```python
from build123d import *

# Parameters (mm, degrees)
F0_R      = 25
F2_DEPTH  = 50
F3_R      = 12.5
F4_DEPTH  = 37.5
F10_D     = 10
F10_DEPTH = 25
F10_TIP   = 3.0043030951
F11_R     = 5
F12_DEPTH = 25


# Not quite as in the source:
# - a feature of the source that left no trace in its solid (it failed there, or was rolled back) is left out


with BuildPart() as f2:
    # F0 (on Top) → F2 (new body)
    with BuildSketch(Plane.XY):
        Circle(F0_R)
    extrude(amount=F2_DEPTH)

    # F3 (on face) → F4 (join)
    with BuildSketch(Plane.XY.offset(50)):
        Circle(F3_R)
    extrude(amount=F4_DEPTH)

    # F10
    with Locations(Plane(origin=(0, 0, 0), x_dir=(1, 0, 0), z_dir=(0, 0, -1))):
        with Locations((0, 0)):
            Hole(F10_D / 2, depth=F10_DEPTH)
            with Locations((0, 0, -(F10_DEPTH + F10_TIP / 2))):  # 118° drill point
                Cone(0, F10_D / 2, F10_TIP, mode=Mode.SUBTRACT)

    # F11 (on face) → F12 (join)
    with BuildSketch(Plane.XY.offset(87.5)):
        Circle(F11_R)
    extrude(amount=F12_DEPTH)


solid = f2.part
```
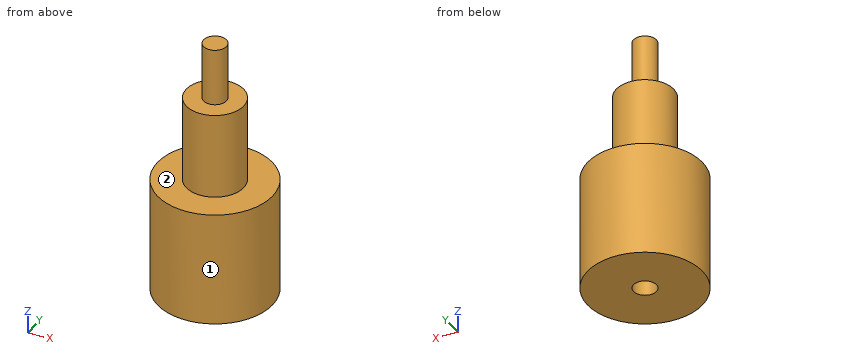
Design review of the part built by this model. Coordinates are the model's own, in mm. Face numbers are marked on the shaded views. A direction names the side the tool comes from. Round coordinates to 2 decimals unless told otherwise and drop trailing zeros. Write each loop counter-clockwise with the first axis right and the second up, starting at its lowest first coordinate (ties: lowest second). Pieces come first, ordered by that corner, then holes. Notation, with made-up numbers: (-17.75, -18) -> (24.25, -18) arc R29 cw to (24.25, 19) -> close; hole circle Ø2 at (10, 65.25). An arc over 180 degrees is marked (long way). Write item = value, one per line. Start each with the question number.
1) Take a section at D-D, the plane z = 43. State the section outline as (x, y) points, plus the area to 3 significant figures.
2) Tool access review of the marked faces 1 and 2: name each direction out of +Z, -Z, +X, -X, +Y, -Y from which nothing blocks a thin tool from reaching the whole face with its end or side.
3) Take a section at A-A, the plane y = -15. State the section outline as (x, z) points, plus the area to 3 significant figures.
4) Wall thickness on probe 1 along Y at (x, z) = (0, 5.75); probe 2 along Z at (x, y) = (15.5, -8.5); probe 3 along Z at (x, y) = (-9, 8.5): over which ranges is each line inside the solid? List them lowest first. Write a range as from..to.
5) Clearance check with flat-ended pins moving along their axes: pin 1 (6 mm diameter, centred on x = -12, z = 25, fed in from -Y); pin 2 (1.5 mm diameter, centred on x = -14, y = -7.5, fed in from +Z); pin 3 (2 mm diameter, centred on x = -1.5, z = 30.5, fed in from -Y) (3 decimals). State where each tip first meets the part, or that it passes through.
6) Take a section at B-B, the plane z = 18. State the section outline as (x, y) points, plus the area to 3 significant figures.
7) Take a section at C-C, the plane x = 6.5. State the section outline as (y, z) points.
Results list:
q1.outline = circle Ø50 at (0, 0)
q1.area = 1,960 mm²
q2.face_1 = +Z, -Z
q2.face_2 = +Z
q3.outline = (-20, 0) -> (20, 0) -> (20, 50) -> (-20, 50) -> close
q3.area = 2,000 mm²
q4.probe_1 = -25..-5, 5..25
q4.probe_2 = 0..50
q4.probe_3 = 0..87.5
q5.pin_1 = -23.32
q5.pin_2 = 50
q5.pin_3 = -24.995
q6.outline = circle Ø50 at (0, 0); hole circle Ø10 at (0, 0)
q6.area = 1,880 mm²
q7.outline = (-24.14, 0) -> (24.14, 0) -> (24.14, 50) -> (10.68, 50) -> (10.68, 87.5) -> (-10.68, 87.5) -> (-10.68, 50) -> (-24.14, 50) -> close
